Autodesk Inventor part; units mm, degrees
ref_plane "YZ Plane" through (0, 0, 0) normal (1, 0, 0) x (0, 1, 0)
ref_plane "XZ Plane" through (0, 0, 0) normal (0, 1, 0) x (-1, 0, 0)
ref_plane "XY Plane" through (0, 0, 0) normal (0, 0, 1) x (1, 0, 0)
sketch "Sketch1" plane through (0, 0, 0) normal (0, 0, 1) x (1, 0, 0)
  line L0 (0, 0) -> (40, 0)
  line L1 (40, 0) -> (40, 40)
  line L2 (40, 40) -> (0, 40)
  line L3 (0, 40) -> (0, 0)
  line L4 (20, 32.5) -> (20, 7.5) construction
  circle A0 centre (20, 32.5) radius 2.5
  circle A1 centre (20, 7.5) radius 2.5
  point P0 (20, 20)
  point P1 (40, 20)
  point P2 (20, 40)
  dimension "d0" = 40
  dimension "d1" = 40
  dimension "d2" = 25
  dimension "d3" = 5
  dimension "d4" = 5
extrude "Extrusion1" add sketch "Sketch1" along normal blind 7
sketch "Sketch2" plane through (0, 0, 7) normal (0, 0, 1) x (1, 0, 0)
  circle A0 centre (20, 32.5) radius 2.5
  circle A1 centre (20, 7.5) radius 2.5
  circle A2 centre (20, 32.5) radius 6.5
  circle A3 centre (20, 7.5) radius 6.5
  point P0 (0, 0)
  dimension "d7" = 13
  dimension "d8" = 13
extrude "Extrusion2" cut sketch "Sketch2" against normal blind 5
sketch "Sketch3" plane through (0, 0, 7) normal (0, 0, 1) x (1, 0, 0)
  circle A0 centre (20, 20) radius 1.5
  line L0 (40, 40) -> (0, 40)
  line L1 (40, 0) -> (40, 40)
  circle A1 centre (24.9497, 24.9497) radius 1.5
  line L2 (20, 20) -> (24.9497, 24.9497) construction
  line L3 (20, 20) -> (27, 20) construction
  circle A2 centre (15.0503, 24.9497) radius 1.5
  circle A3 centre (15.0503, 15.0503) radius 1.5
  circle A4 centre (24.9497, 15.0503) radius 1.5
  point P0 (0, 0)
  point P1 (20, 40)
  point P2 (40, 20)
  dimension "d11" = 3
  dimension "d12" = 3
  dimension "d13" = 45
  dimension "d14" = 7
  dimension "d17" = 360
extrude "Extrusion3" cut sketch "Sketch3" against normal through all
fillet "Fillet1" radius 10 4 edges at (40, 40, 3.5) (40, 0, 3.5) (0, 40, 3.5) (0, 0, 3.5)
properties part number "AA047" material "ABS Plastic"
Work out the finished part from the listing and answer in its coordinate system (mm). A direction names the side the tool comes from. Round coordinates to 2 decimals unless told otherwise and drop trailing zeros. Write each loop counter-clockwise with the first axis right and the second up, starting at its lowest first coordinate (ties: lowest second). Pieces come first, ordered by that corner, then holes. Notation, with made-up numbers: (58, 62) - (104, 62) arc R12 ccw to (104, 66) - close; hole circle Ø11 at (5.25, 21.5). An arc over 180 degrees is marked (long way). Return JSON: item names as keys, results as strings. Group by question number.
Q1. The part is cut by section A-A on x = 20. Write down the section's boundary in (y, z).
Q2. Find the intervals of material crossed by L1, parallel to Y at x = 20, z = 0.65; L2, parallel to X at y = 10, z = 5.5; L3, parallel to Y at x = 19, z = 2.75, in increasing order.
Q3. The part is cut by section D-D on x = 16. Write down the section's boundary in (y, z).
Q4. The part is cut by section B-B on y = 20. Write down the section's boundary in (x, z).
Q5. Each of these flat-tipped pins is pushed along its axis until it touches: pin 1 Ø1 at (y, z) = (18, 4) entering from -X; pin 2 Ø4 at (x, y) = (20, 7.5) entering from +Z; pin 3 Ø6.5 at (x, y) = (22, 33.5) entering from +Z; pin 4 Ø3 at (x, z) = (34, 2) entering from -Y. Where does it stop, or does it pass through?
Q6. The mould has two halves that part along Y. Classify faces 3 (the cylindrical face through (17.5, 7.4, 1)), 4 (the flat face through (20, 40, 3)), 5 (the flat face through (20, 0, 3)): released by +Y, released by -Y, zero draft, split by the parting line, or undercut.
Q7. For faces 1 (the flat face through (23, 33, 2)), 2 (the flat face through (15, 20, 7)), determine the directions among +Z, -Z, +X, -X, +Y, -Y from which every point of the face is accessible in a straight line to the end or side of a thin tool.
Q8. The part is cut by section C-C on z = 4. Write down the section's boundary in (x, y), then the cut area to 3 significant figures.
Solved:
{
 "1": {"outline": "(0, 0) - (5, 0) - (5, 2) - (1, 2) - (1, 7) - (0, 7) - close; (10, 0) - (18.5, 0) - (18.5, 7) - (14, 7) - (14, 2) - (10, 2) - close; (21.5, 0) - (30, 0) - (30, 2) - (26, 2) - (26, 7) - (21.5, 7) - close; (35, 0) - (40, 0) - (40, 7) - (39, 7) - (39, 2) - (35, 2) - close"},
 "2": {"L1": "0 to 5, 10 to 18.5, 21.5 to 30, 35 to 40", "L2": "0 to 14, 26 to 40", "L3": "0 to 1.08, 13.92 to 18.88, 21.12 to 26.08, 38.92 to 40"},
 "3": {"outline": "(0, 0) - (13.89, 0) - (13.89, 7) - (12.62, 7) - (12.62, 2) - (2.38, 2) - (2.38, 7) - (0, 7) - close; (16.21, 0) - (23.79, 0) - (23.79, 7) - (16.21, 7) - close; (26.11, 0) - (40, 0) - (40, 7) - (37.62, 7) - (37.62, 2) - (27.38, 2) - (27.38, 7) - (26.11, 7) - close"},
 "4": {"outline": "(0, 0) - (18.5, 0) - (18.5, 7) - (0, 7) - close; (21.5, 0) - (40, 0) - (40, 7) - (21.5, 7) - close"},
 "5": {"pin 1": "x = 0", "pin 2": "through", "pin 3": "z = 2", "pin 4": "y = 0.32"},
 "6": {"face 3": "undercut", "face 4": "released by +Y", "face 5": "released by -Y"},
 "7": {"face 1": "+Z", "face 2": "+Z, +X, -X, +Y, -Y"},
 "8": {"outline": "(0, 10) arc R10 ccw to (10, 0) - (30, 0) arc R10 ccw to (40, 10) - (40, 30) arc R10 ccw to (30, 40) - (10, 40) arc R10 ccw to (0, 30) - close; hole circle Ø13 at (20, 7.5); hole circle Ø13 at (20, 32.5); hole circle Ø3 at (15.05, 15.05); hole circle Ø3 at (15.05, 24.95); hole circle Ø3 at (20, 20); hole circle Ø3 at (24.95, 15.05); hole circle Ø3 at (24.95, 24.95)", "area": "1,210 mm²"}
}
